Autodesk Inventor part; units mm, degrees
ref_plane "YZ Plane" through (0, 0, 0) normal (1, 0, 0) x (0, 1, 0)
ref_plane "XZ Plane" through (0, 0, 0) normal (0, 1, 0) x (-1, 0, 0)
ref_plane "XY Plane" through (0, 0, 0) normal (0, 0, 1) x (1, 0, 0)
sketch "Sketch8" plane through (0, 0, 0) normal (0, 1, 0) x (-1, 0, 0)
  circle A0 centre (0, 0) radius 6.35
  point P0 (0, 0)
extrude "Extrusion4" add sketch "Sketch8" against normal blind 55
chamfer "Chamfer2" distance 1.27 angle 45 1 edges at (6.35, -55, 0)
sketch "Sketch9" plane through (0, 0, 0) normal (0, 0, 1) x (1, 0, 0)
  line L0 (-6.35, 0) -> (-6.35, -53.73)
  line L1 (-4.7625, -22.225) -> (-4.7625, -23.8125)
  line L2 (-6.35, -25.4) -> (-6.35, -20.6375)
  line L3 (-6.35, -41.275) -> (-4.7625, -41.275)
  line L4 (-4.7625, -41.275) -> (-4.7625, -39.6875)
  line L5 (-4.7625, -39.6875) -> (-6.35, -39.6875)
  line L6 (-6.35, -39.6875) -> (-6.35, -41.275)
  line L7 (0, -64.476) -> (0, 10.746)
  line L8 (-4.7625, -22.225) -> (-6.35, -20.6375)
  line L9 (-4.7625, -23.8125) -> (-6.35, -25.4)
  point P0 (0, 0)
revolve "Revolution1" cut sketch "Sketch9" angle 360 about axis through (0, -10, 0) along (0, 1, 0)
properties part number "Crank shaft" material "Steel, High Strength Low Alloy"
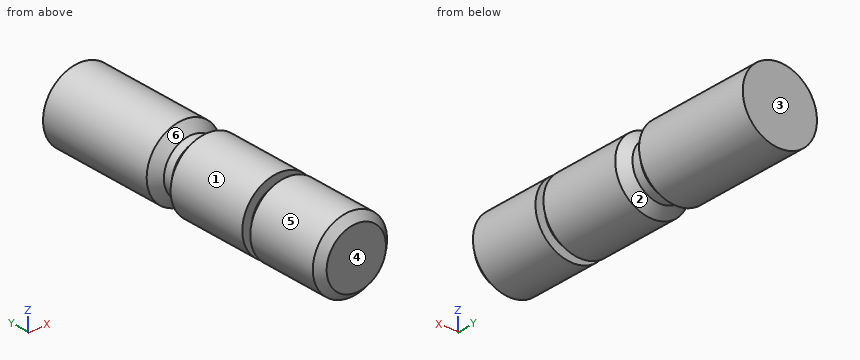
Work out the finished part from the listing and answer in its coordinate system (mm). Face numbers are marked on the shaded views. A direction names the side the tool comes from. Give positions to 0.01 mm unless a question says otherwise; leave off trailing zeros. Loops run counter-clockwise (first coordinate to the right, second up) from the corner with the lowest first, then second, coordinate; pieces in that order, holes last. Notation, with made-up numbers: (-7.5, -21) -> (12.5, -21) arc R24 ccw to (12.5, 9) -> close; hole circle Ø2 at (0, 14). An arc over 180 degrees is marked (long way). Use a Markdown table: item, result. Add a question column.
1. Determine the mould class of the marked faces 1, 2, 3 and 4 for opening direction Y: released by +Y, released by -Y, zero draft, split by the parting line, or undercut.
2. Section C-C on y = -3.5 is taken. Determine the outline of the cut face in (x, z).
3. Find the intervals of material crossed by probe 1 along Y at (x, z) = (-1.5, 5) (1 decimal); probe 2 along Y at (x, z) = (1.75, 4.75) (1 decimal); probe 3 along X at (y, z) = (-43, -1.5), in increasing order.
4. For the marked faces 5 and 6, determine the directions among +Z, -Z, +X, -X, +Y, -Y from which every point of the face is accessible in a straight line to the end or side of a thin tool.
5. Flat-ended cylindrical pins translate along their axes: pin 1 Ø1 at (y, z) = (-28, -2.5) entering from -X; pin 2 Ø5 at (y, z) = (-23, 4) entering from -X; pin 3 Ø4 at (y, z) = (-26.5, 2.5) entering from +X. Find the tip coordinate at first contact, or state that the pin passes through.
Results below:
| question | item | result |
|---|---|---|
| 1 | face 1 | zero draft |
| 1 | face 2 | undercut |
| 1 | face 3 | released by +Y |
| 1 | face 4 | released by -Y |
| 2 | outline | circle Ø12.7 at (0, 0) |
| 3 | probe 1 | y = -54.9 to -41.3, -39.7 to -24.3, -21.8 to 0 |
| 3 | probe 2 | y = -55 to -41.3, -39.7 to -24.1, -21.9 to 0 |
| 3 | probe 3 | x = -6.17 to 6.17 |
| 4 | face 5 | +Y, -Y |
| 4 | face 6 | none |
| 5 | pin 1 | stops at x = -6.03 |
| 5 | pin 2 | stops at x = -5.52 |
| 5 | pin 3 | stops at x = 6.33 |
